```python
from build123d import *

# Parameters (mm, degrees)
SKETCH_1_R          = 1.6
EXTRUDE_1_DEPTH     = 10
SKETCH_2_W          = 19.899365944
SKETCH_2_H          = 5
CUT_EXTRUDE_1_DEPTH = 10
FILLET_1_R          = 1


with BuildPart() as part:
    # 草图1 → 凸台-拉伸1 (new body)
    with BuildSketch(Plane(origin=(0, 0, 0), x_dir=(1, 0, 0), z_dir=(0, 1, 0))):
        with BuildLine():
            Line((-4, 0), (-4, 20))
            ThreePointArc((-4, 20), (0, 24), (4, 20))
            Line((4, 20), (4, 0))
            ThreePointArc((4, 0), (0, -4), (-4, 0))
        make_face()
        with Locations((0, 20)):
            Circle(SKETCH_1_R, mode=Mode.SUBTRACT)
        Circle(SKETCH_1_R, mode=Mode.SUBTRACT)
    extrude(amount=EXTRUDE_1_DEPTH)

    # 草图2 → 切除-拉伸1 (cut)
    with BuildSketch(Plane(origin=(4, 0, 0), x_dir=(0, 0, -1), z_dir=(1, 0, 0))):
        with Locations((0, 5)):
            Rectangle(SKETCH_2_W, SKETCH_2_H)
    extrude(amount=-CUT_EXTRUDE_1_DEPTH, mode=Mode.SUBTRACT)

    # 圆角1
    fillet_1_edges = [part.edges().sort_by_distance(p)[0] for p in [
        (4, 10, -10),
        (0, 10, -24),
        (-4, 5, -9.949682972),
        (-4, 10, -10),
        (4, 5, -9.949682972),
        (0, 10, 4),
        (0, 0, 4),
        (-4, 0, -10),
        (0, 0, -24),
        (4, 0, -10),
    ]]
    fillet(fillet_1_edges, radius=FILLET_1_R)


solid = part.part
```
Part model, mm, in its own coordinate system. A direction names the side the tool comes from. Give positions to 0.01 mm unless a question says otherwise; leave off trailing zeros. Write each loop counter-clockwise with the first axis right and the second up, starting at its lowest first coordinate (ties: lowest second). Pieces come first, ordered by that corner, then holes. Notation, with made-up numbers: (-29.5, -23.75) -> (7.5, -23.75) arc R35 cw to (7.5, 10.25) -> close; hole circle Ø9 at (75.25, 2). An arc over 180 degrees is marked (long way). Put each result on its own line as item: value. Start each with the question number.
Item 1: Cut at C-C (y = 7.25). List the corners of the cut face in (x, z), then the cut area to 3 significant figures.
Item 2: Cut at A-A (z = -8.5). List the corners of the cut face in (x, y), then the cut area to 3 significant figures.
Item 3: Wall check: L1, parallel to Z at x = 0, y = 8.4; L2, parallel to Y at x = 2.25, z = -1.5; L3, parallel to X at y = 8.35, z = 0. Give the ranges that are in metal, low to high. Write a range as [from, to].
Item 4: Pin check, flat tip, straight feed: pin 1 Ø3 at (x, y) = (-3, 3) entering from +Z. Stop position of the tip, or through.
Item 5: Pull direction Z, two halves, no side cores. Call faces 4 (the face through (0, 5, -24)), 5 (the face through (-1.27, 1.23, 0.97)), 6 (the face through (0, 2.5, -3)): pulls with the +Z half, pulls with the -Z half, needs draft (parallel to the pull), parting line crosses it, or undercut.
Item 6: Cut at B-B (x = 0). List the corners of the cut face in (y, z).
Item 7: Which spindle directions (+Z, -Z, +X, -X, +Y, -Y) get a long thin tool onto all of the face, cutting with end or side? Do faces 1 (the face through (3.699, 0.285, -9.86)), 2 (the face through (-3.715, 4.965, -10.25)), 3 (the face through (3.699, 5.035, -10.235)). Say none if no direction does.
Answer list:
1. outline: (-4, -20) arc R4 ccw to (4, -20) -> (4, -10.95) arc R1 ccw to (3, -9.95) -> (-3, -9.95) arc R1 ccw to (-4, -10.95) -> close; hole circle Ø3.2 at (0, -20)
1. area: 97.1 mm2
2. outline: (-4, 1) arc R1 ccw to (-3, 0) -> (3, 0) arc R1 ccw to (4, 1) -> (4, 2.5) -> (-4, 2.5) -> close; (-4, 7.5) -> (4, 7.5) -> (4, 9) arc R1 ccw to (3, 10) -> (-3, 10) arc R1 ccw to (-4, 9) -> close
2. area: 39.1 mm2
3. L1: z = [-24, -21.6], [-18.4, -1.6], [1.6, 4]
3. L2: y = [0, 2.5], [7.5, 10]
3. L3: x = [-4, -1.6], [1.6, 4]
4. pin 1: stops at z = 3.67
5. face 4: pulls with the -Z half
5. face 5: undercut
5. face 6: needs draft
6. outline: (0, -23) arc R1 ccw to (1, -24) -> (9, -24) arc R1 ccw to (10, -23) -> (10, -21.6) -> (0, -21.6) -> close; (0, -18.4) -> (10, -18.4) -> (10, -1.6) -> (7.5, -1.6) -> (7.5, -9.95) -> (2.5, -9.95) -> (2.5, -1.6) -> (0, -1.6) -> close; (0, 1.6) -> (2.5, 1.6) -> (2.5, 4) -> (1, 4) arc R1 ccw to (0, 3) -> close; (7.5, 1.6) -> (10, 1.6) -> (10, 3) arc R1 ccw to (9, 4) -> (7.5, 4) -> close
7. face 1: +Z, -Z, +X, -Y
7. face 2: +Z, -X
7. face 3: +Z, +X
